```python
from build123d import *

# Parameters (mm, degrees)
F0_R     = 90.17
F0_R_2   = 66.675
F1_DEPTH = 12.7
F2_R     = 2.2225
F3_DEPTH = 12.701
F5_DEPTH = 12.701


with BuildPart() as f1:
    # F0 (on Front) → F1 (new body)
    with BuildSketch(Plane.XZ):
        Circle(F0_R)
        Circle(F0_R_2, mode=Mode.SUBTRACT)
    extrude(amount=F1_DEPTH)

    # F2 (on face) → F3 (cut, through all)
    with BuildSketch(Plane.XZ.offset(12.7)):
        with Locations((-58.42, 58.42)):
            Circle(F2_R)
        with Locations((-50.165, 50.165)):
            Circle(F2_R)
        with Locations((50.165, 50.165)):
            Circle(F2_R)
        with Locations((58.42, 58.42)):
            Circle(F2_R)
        with Locations((50.165, -50.165)):
            Circle(F2_R)
        with Locations((58.42, -58.42)):
            Circle(F2_R)
        with Locations((-58.42, -58.42)):
            Circle(F2_R)
        with Locations((-50.165, -50.165)):
            Circle(F2_R)
    extrude(amount=-F3_DEPTH, mode=Mode.SUBTRACT)

    # F4 (on face) → F5 (cut, through all)
    with BuildSketch(Plane.XZ.offset(12.7)):
        with BuildLine():
            Line((15.875, 69.85), (-15.875, 69.85))
            Line((-15.875, 69.85), (-15.875, 64.757548))
            ThreePointArc((-15.875, 64.757548), (0, 66.675), (15.875, 64.757548))
            Line((15.875, 64.757548), (15.875, 69.85))
        make_face()
    extrude(amount=-F5_DEPTH, mode=Mode.SUBTRACT)


solid = f1.part
```
Verification items for the finished model (mm, model axes). A direction names the side the tool comes from. Coordinates: 2 decimals unless noted, no trailing zeros. Loops run counter-clockwise (first coordinate to the right, second up) from the corner with the lowest first, then second, coordinate; pieces in that order, holes last. Notation, with made-up numbers: (-15.5, -28.5) -> (10.5, -28.5) arc R16 cw to (10.5, -6.5) -> close; hole circle Ø11 at (-9.5, 84.5). An arc over 180 degrees is marked (long way). Answer in a Markdown table with one row per item. Add a question column.
1. Section check B-B, the plane z = -28. Enter the section's corners in (x, y), then the cut area to 3 significant figures.
2. Section check C-C, the plane y = -8. Give the number of separate pieces and of enclosed holes in the cut face, then the cut area to 3 significant figures.
3. Section check A-A, the plane x = 0. Enter the section's corners in (y, z) (3 decimals).
4. Depth check by flat-ended pin: P1, Ø3.5, axis at x = 50.165, z = -50.165, coming from the -Y side; P2, Ø2.5, axis at y = -7, z = 67, coming from the -X side; P3, Ø7, axis at x = -50.165, z = 50.165, coming from the +Y side; P4, Ø3, axis at x = 68, y = -5, coming from the +Z side. Enter the tip coordinate at first touch or a pass-through.
5. Access from +Z, -Z, +X, -X, +Y, -Y to the whole of each face (thin tool, end or side, straight path). Record for faces 4 (the face through (15.875, -6, 67)), 5 (the face through (-67, -12.7, 0)).
6. Section check D-D, the plane z = -58.42. Enter the section's corners in (x, y), then the cut area to 3 significant figures.
7. Draft check along Z on faces 1 (the face through (-50.647, -6.439, -52.335)), 2 (the face through (-67, 0, 0)), 3 (the face through (-19.547, -6.261, -88.026)). Enter one of: +Z half, -Z half, draft (parallel to the pull), parting line (faces both ways), or undercut.
8. Material ranges on probe 1 along X at (y, z) = (-10, -58.5); probe 2 along Z at (x, y) = (-58.42, -3.5); probe 3 along Z at (x, y) = (51.5, -8.5), recorded low to high. Write a range as [from, to].
Derived:
| question | item | result |
|---|---|---|
| 1 | outline | (-85.71, -12.7) -> (-60.51, -12.7) -> (-60.51, 0) -> (-85.71, 0) -> close; (60.51, -12.7) -> (85.71, -12.7) -> (85.71, 0) -> (60.51, 0) -> close |
| 1 | area | 640 mm² |
| 2 | separate pieces | 1 |
| 2 | enclosed holes | 9 |
| 2 | area | 11,300 mm² |
| 3 | outline | (-12.7, -90.17) -> (0, -90.17) -> (0, -66.675) -> (-12.7, -66.675) -> close; (-12.7, 69.85) -> (0, 69.85) -> (0, 90.17) -> (-12.7, 90.17) -> close |
| 4 | P1 | passes through |
| 4 | P2 | stops at x = -61.71 |
| 4 | P3 | stops at y = 0 |
| 4 | P4 | stops at z = 60.9 |
| 5 | face 4 | +Y, -Y |
| 5 | face 5 | +Z, -Z, +X, -X, -Y |
| 6 | outline | (-68.69, -12.7) -> (-60.64, -12.7) -> (-60.64, 0) -> (-68.69, 0) -> close; (-56.2, -12.7) -> (-32.14, -12.7) -> (-32.14, 0) -> (-56.2, 0) -> close; (32.14, -12.7) -> (56.2, -12.7) -> (56.2, 0) -> (32.14, 0) -> close; (60.64, -12.7) -> (68.69, -12.7) -> (68.69, 0) -> (60.64, 0) -> close |
| 6 | area | 815 mm² |
| 7 | face 1 | undercut |
| 7 | face 2 | draft |
| 7 | face 3 | parting line |
| 8 | probe 1 | x = [-68.62, -60.64], [-56.2, -31.99], [31.99, 56.2], [60.64, 68.62] |
| 8 | probe 2 | z = [-68.69, -60.64], [-56.2, -32.14], [32.14, 56.2], [60.64, 68.69] |
| 8 | probe 3 | z = [-74.02, -51.94], [-48.39, -42.35], [42.35, 48.39], [51.94, 74.02] |
